```python
from build123d import *

# Parameters (mm, degrees)
F1_DEPTH = 12.7


with BuildPart() as f1:
    # F0 (on Top) → F1 (new body)
    with BuildSketch(Plane.XY):
        with BuildLine():
            Line((-11.216301, 6.446693), (-11.216301, 0))
            Line((-11.216301, 0), (16.996317, 0))
            Line((16.996317, 0), (16.996317, 6.446693))
            Line((16.996317, 6.446693), (15.065662, 6.446693))
            ThreePointArc((15.065662, 6.446693), (11.193809, 2.90156), (7.321957, 6.446693))
            Line((7.321957, 6.446693), (0, 6.446693))
            ThreePointArc((0, 6.446693), (-3.892248, 2.668559), (-7.784497, 6.446693))
            Line((-7.784497, 6.446693), (-11.216301, 6.446693))
        make_face()
    extrude(amount=F1_DEPTH)


solid = f1.part
```
Design review of the part built by this model. Coordinates are the model's own, in mm. Give positions to 0.01 mm unless a question says otherwise; leave off trailing zeros. Loops run counter-clockwise (first coordinate to the right, second up) from the corner with the lowest first, then second, coordinate; pieces in that order, holes last. Notation, with made-up numbers: M 66.5,9.25 L 92.5,9.25 A19 ccw 92.5,26.25 Z; hole C 74.5,-38 d3. An arc over 180 degrees is marked long. Return JSON: item names as keys, results as strings. Group by question number.
Item 1: Mouldability with a two-part tool opening along X and no side actions: class faces 1 (the cylindrical face through (11.274, 2.902, 6.261)), 2 (the flat face through (-11.216, 3, 6)), 3 (the flat face through (4, 6.447, 6)), 4 (the cylindrical face through (-3.81, 2.67, 6.26)) as released by +X, released by -X, zero draft, split by the parting line, or undercut.
Item 2: We need section A-A (y = 3.25). Give the boundary of the cut face in (x, z), and give its area (3 significant figures).
Item 3: We need section D-D (x = 14.5). Give the boundary of the cut face in (y, z), and give its area (3 significant figures).
Item 4: We need section B-B (z = 7). Give the boundary of the cut face in (x, y).
Item 5: For probe 1 along X at (y, z) = (5, 0.5); probe 2 along X at (y, z) = (6.25, 10.5); probe 3 along Y at (x, z) = (11.25, 1.75), list the stretches that pass through material, from the lowest coordinate up.
Item 6: We need section C-C (y = 5). Give the boundary of the cut face in (x, z), and give its area (3 significant figures).
Item 7: Insertion check: pin 1 Ø2 at (x, z) = (11, 2.5) entering from +Y. The pin has a flat end and moves straight along its axis. Give the tip position at first contact, or say it passes through.
Output:
{
 "1": {"face 1": "undercut", "face 2": "released by -X", "face 3": "zero draft", "face 4": "undercut"},
 "2": {"outline": "M -11.22,0 L -5.94,0 L -5.94,12.7 L -11.22,12.7 Z; M -1.85,0 L 9.59,0 L 9.59,12.7 L -1.85,12.7 Z; M 12.8,0 L 17,0 L 17,12.7 L 12.8,12.7 Z", "area": "265 mm^2"},
 "3": {"outline": "M 0,0 L 4.74,0 L 4.74,12.7 L 0,12.7 Z", "area": "60.3 mm^2"},
 "4": {"outline": "M -11.22,0 L 17,0 L 17,6.45 L 15.07,6.45 A3.89 cw 7.32,6.45 L 0,6.45 A3.89 cw -7.78,6.45 L -11.22,6.45 Z"},
 "5": {"probe 1": "x = -11.22 to -7.46, -0.33 to 7.74, 14.64 to 17", "probe 2": "x = -11.22 to -7.77, -0.01 to 7.34, 15.04 to 17", "probe 3": "y = 0 to 2.9"},
 "6": {"outline": "M -11.22,0 L -7.46,0 L -7.46,12.7 L -11.22,12.7 Z; M -0.33,0 L 7.74,0 L 7.74,12.7 L -0.33,12.7 Z; M 14.64,0 L 17,0 L 17,12.7 L 14.64,12.7 Z", "area": "180 mm^2"},
 "7": {"pin 1": "stops at y = 3.09"}
}
